Check sheet for the drawn part. Datum: minimum x, y, z corner. Units: mm. A direction names the side the tool comes from. Round coordinates to 2 decimals unless told otherwise and drop trailing zeros. Order: outer loops, then holes, each group sorted by start corner. A loop starts at its lowest first (then second) coordinate and runs counter-clockwise, first axis right, second up. Notation, with made-up numbers: (-9.5, -35.75) -> (19.5, -35.75) arc R19 cw to (19.5, -29.75) -> close; hole circle Ø9 at (-29, 61.25). An arc over 180 degrees is marked (long way). Answer in a Markdown table with one row per item.
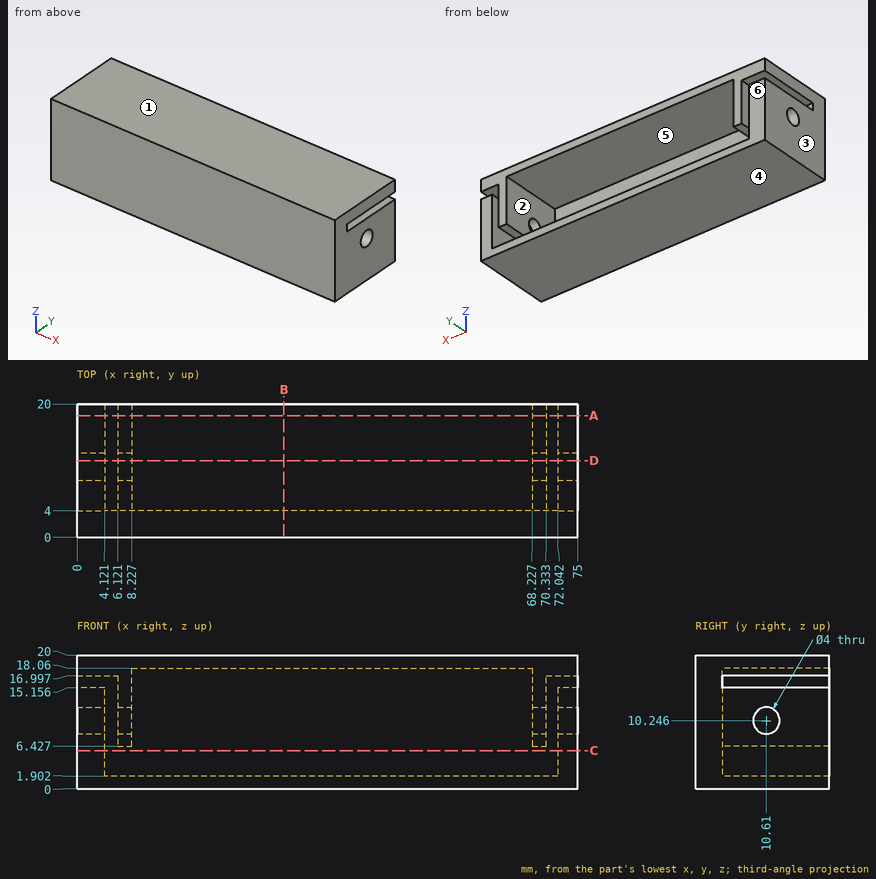
(1) Section check D-D on y = 11.5. Give the number of separate pieces and of enclosed holes in the cut face, plus the area to 3 significant figures.
Solutions:
| item | result |
|---|---|
| separate pieces | 6 |
| enclosed holes | 0 |
| area | 402 mm^2 |
(2) Section check B-B on x = 31. Record the boundary of the cut face in (y, z).
Solutions:
| item | result |
|---|---|
| outline | (0, 0) -> (20, 0) -> (20, 1.9) -> (4, 1.9) -> (4, 18.06) -> (20, 18.06) -> (20, 20) -> (0, 20) -> close |
(3) Draft check along Z on the marked faces 1, 2, 3 and 4. Enter one of: pulls with the +Z half, pulls with the -Z half, needs draft (parallel to the pull), parting line crosses it, or undercut.
Solutions:
| item | result |
|---|---|
| face 1 | pulls with the +Z half |
| face 2 | undercut |
| face 3 | needs draft |
| face 4 | pulls with the -Z half |
(4) Tool access check on the marked faces 5 and 6. Record the directions out of +Z, -Z, +X, -X, +Y, -Y that give a thin tool (end or side, any length) a straight path to the whole face; none if there is none.
Solutions:
| item | result |
|---|---|
| face 5 | +Y |
| face 6 | +Z, -Z, +X, -X, +Y |
(5) Section check A-A on y = 18.25. Record the boundary of the cut face in (x, z).
Solutions:
| item | result |
|---|---|
| outline | (0, 0) -> (75, 0) -> (75, 15.16) -> (72.04, 15.16) -> (72.04, 1.9) -> (4.12, 1.9) -> (4.12, 15.16) -> (0, 15.16) -> close; (0, 17) -> (6.12, 17) -> (6.12, 6.43) -> (8.23, 6.43) -> (8.23, 18.06) -> (68.23, 18.06) -> (68.23, 6.43) -> (70.33, 6.43) -> (70.33, 17) -> (75, 17) -> (75, 20) -> (0, 20) -> close |
(6) Scan lines: probe 1 along X at (y, z) = (11.5, 13.5); probe 2 along Z at (x, y) = (65.5, 14.25); probe 3 along X at (y, z) = (4.25, 3.5). Record each from-to range of solid material in increasing order. Write a range as from..to.
Solutions:
| item | result |
|---|---|
| probe 1 | 0..4.12, 6.12..8.23, 68.23..70.33, 72.04..75 |
| probe 2 | 0..1.9, 18.06..20 |
| probe 3 | 0..4.12, 72.04..75 |
(7) Section check C-C on z = 5.75. Record the boundary of the cut face in (x, y), plus the area to 3 significant figures.
Solutions:
| item | result |
|---|---|
| outline | (0, 0) -> (75, 0) -> (75, 20) -> (72.04, 20) -> (72.04, 4) -> (4.12, 4) -> (4.12, 20) -> (0, 20) -> close |
| area | 413 mm^2 |
